Build history of the part. All positions in model axes, mm. Round coordinates to 2 decimals unless told otherwise and drop trailing zeros. Loops run counter-clockwise (first coordinate to the right, second up) from the corner with the lowest first, then second, coordinate; pieces in that order, holes last. Notation, with made-up numbers: (10.25, 68.5) - (65.25, 68.5) arc R16 ccw to (65.25, 93.5) - close; hole circle Ø3 at (-25.5, 59.25). An arc over 180 degrees is marked (long way). Use one line per item in the form item = value. Start each with the question number.
Q1. Drill centre lines: line 1 (Y direction, x = -28.5, z = 3.2); line 2 (X direction, y = -67, z = 3.8); line 3 (X direction, y = 30, z = 3.35). Where is each one in solid material? Low to high.
Q2. Saw through at B-B (z = 3.05). Give the cut face in (x, y), then the cut area to 3 significant figures.
Q3. Saw through at C-C (y = 39). Give the cut face in (x, z).
Q4. Saw through at A-A (x = 14.5). Give the cut face in (y, z).
Q5. Pin check, flat tips, straight feed: pin 1 (2.5 mm diameter, centred on y = -71.5, z = 3, fed in from +X); pin 2 (2.5 mm diameter, centred on x = -20.5, z = 3.5, fed in from -Y). Stop position of each tip, or through.
Q6. Saw through at D-D (x = -54). Give the cut face in (y, z).
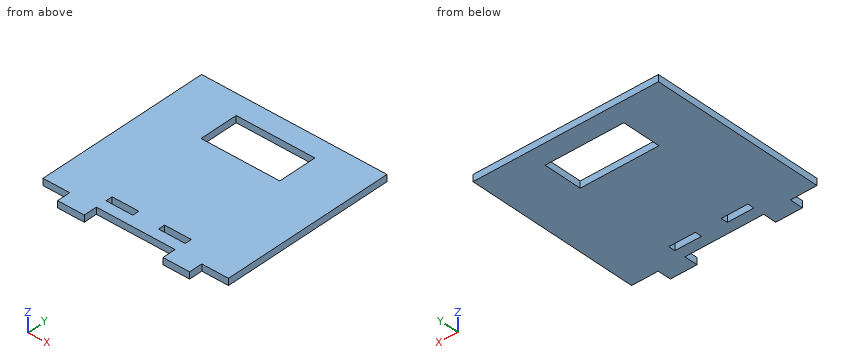
```python
from build123d import *

# Parameters (mm, degrees)
SKETCH1_W           = 139
SKETCH1_H           = 131
SKETCH1_W_2         = 20
SKETCH1_H_2         = 5
SKETCH1_W_3         = 59
SKETCH1_H_3         = 29
SKETCH1_H_4         = 10
BOSS_EXTRUDE2_DEPTH = 5


with BuildPart() as part:
    # Sketch1 → Boss-Extrude2 (new body)
    with BuildSketch(Plane.XY):
        Rectangle(SKETCH1_W, SKETCH1_H)
        with Locations((-19.5, -55)):
            Rectangle(SKETCH1_W_2, SKETCH1_H_2, mode=Mode.SUBTRACT)
        with Locations((19.819504059, -55)):
            Rectangle(SKETCH1_W_2, SKETCH1_H_2, mode=Mode.SUBTRACT)
        with Locations((0, 35.5)):
            Rectangle(SKETCH1_W_3, SKETCH1_H_3, mode=Mode.SUBTRACT)
        with Locations((-39.5, -70.5)):
            Rectangle(SKETCH1_W_2, SKETCH1_H_4)
        with Locations((39.5, -70.5)):
            Rectangle(SKETCH1_W_2, SKETCH1_H_4)
    extrude(amount=BOSS_EXTRUDE2_DEPTH)


solid = part.part
```
Report:
q1.line_1 = -65.5 to -57.5, -52.5 to 21, 50 to 65.5
q1.line_2 = -49.5 to -29.5, 29.5 to 49.5
q1.line_3 = -69.5 to -29.5, 29.5 to 69.5
q2.outline = (-69.5, -65.5) - (-49.5, -65.5) - (-49.5, -75.5) - (-29.5, -75.5) - (-29.5, -65.5) - (29.5, -65.5) - (29.5, -75.5) - (49.5, -75.5) - (49.5, -65.5) - (69.5, -65.5) - (69.5, 65.5) - (-69.5, 65.5) - close; hole (-29.5, -57.5) - (-9.5, -57.5) - (-9.5, -52.5) - (-29.5, -52.5) - close; hole (-29.5, 21) - (29.5, 21) - (29.5, 50) - (-29.5, 50) - close; hole (9.82, -57.5) - (29.82, -57.5) - (29.82, -52.5) - (9.82, -52.5) - close
q2.area = 16,700 mm²
q3.outline = (-69.5, 0) - (-29.5, 0) - (-29.5, 5) - (-69.5, 5) - close; (29.5, 0) - (69.5, 0) - (69.5, 5) - (29.5, 5) - close
q4.outline = (-65.5, 0) - (-57.5, 0) - (-57.5, 5) - (-65.5, 5) - close; (-52.5, 0) - (21, 0) - (21, 5) - (-52.5, 5) - close; (50, 0) - (65.5, 0) - (65.5, 5) - (50, 5) - close
q5.pin_1 = 49.5
q5.pin_2 = -65.5
q6.outline = (-65.5, 0) - (65.5, 0) - (65.5, 5) - (-65.5, 5) - close
